Geometry: see drawing. Coordinates: mm, zero at the bounding-box minimum. Give positions to 0.01 mm unless a question says otherwise; leave off trailing zeros. Loops run counter-clockwise (first coordinate to the right, second up) from the corner with the lowest first, then second, coordinate; pieces in that order, holes last. Notation, with made-up numbers: M -17,-25 L 41,-25 A19 ccw 41,-16 Z; hole C -34.5,85 d6. An arc over 180 degrees is marked long. Use CSV: the item, a comma, the result in double quotes. Start each with the question number.
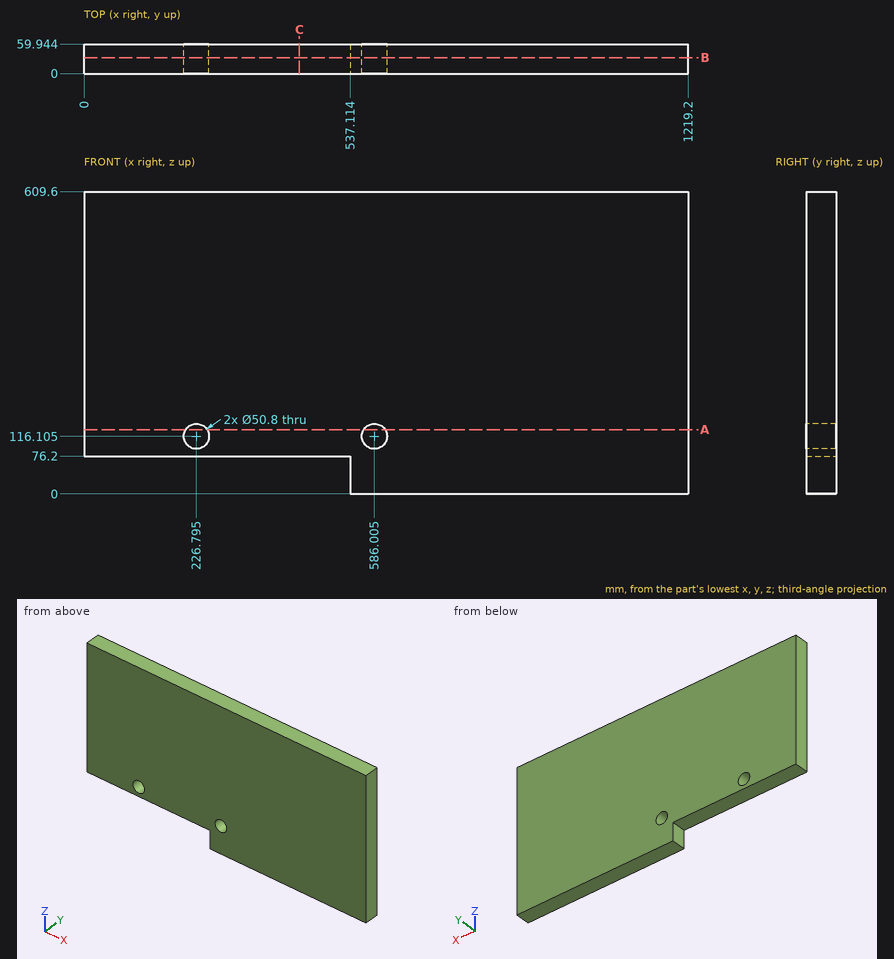
Item 1: Material intervals for line 1 (X direction, y = 13, z = 115.5); line 2 (X direction, y = 6, z = 94) (1 decimal); line 3 (Z direction, x = 331, y = 32.5), sorted ascending.
Item 2: Section B-B (y = 32.5). Output: boundary loops of the cut face in (x, z) (1 decimal), then the cut area to 3 significant figures.
Item 3: First-contact query: pin 1 Ø12 at (x, y) = (475, 45.5) entering from -Z. Flat tip, straight axial feed; report the tip coordinate or a pass-through.
Item 4: Section C-C (x = 434.5). Output: boundary loops of the cut face in (y, z).
Item 5: Section A-A (z = 129.5). Output: boundary loops of the cut face in (x, y) (1 decimal).
Recorded:
1,line 1,"0 to 201.4, 252.19 to 560.61, 611.4 to 1219.2"
1,line 2,"0 to 214.3, 239.3 to 573.5, 598.5 to 1219.2"
1,line 3,"76.2 to 609.6"
2,outline,"M 0,76.2 L 537.1,76.2 L 537.1,0 L 1219.2,0 L 1219.2,609.6 L 0,609.6 Z; hole C 226.8,116.1 d50.8; hole C 586,116.1 d50.8"
2,area,"698,000 mm²"
3,pin 1,"z = 76.2"
4,outline,"M 0,76.2 L 59.94,76.2 L 59.94,609.6 L 0,609.6 Z"
5,outline,"M 0,0 L 205.2,0 L 205.2,59.9 L 0,59.9 Z; M 248.4,0 L 564.4,0 L 564.4,59.9 L 248.4,59.9 Z; M 607.6,0 L 1219.2,0 L 1219.2,59.9 L 607.6,59.9 Z"
